Print and shaded views of the part. All mm, measured from the part's lowest x, y and z. A direction names the side the tool comes from. Give positions to 0.01 mm unless a question says otherwise; leave off trailing zeros. Loops run counter-clockwise (first coordinate to the right, second up) from the corner with the lowest first, then second, coordinate; pieces in that order, holes last. Notation, with made-up numbers: (39, 42) -> (79, 42) arc R24 ccw to (79, 80) -> close; hole circle Ø1 at (81, -18). An arc over 180 degrees is marked (long way). Write each question's results on one line, items separated by ' | '. Start each with the question number.
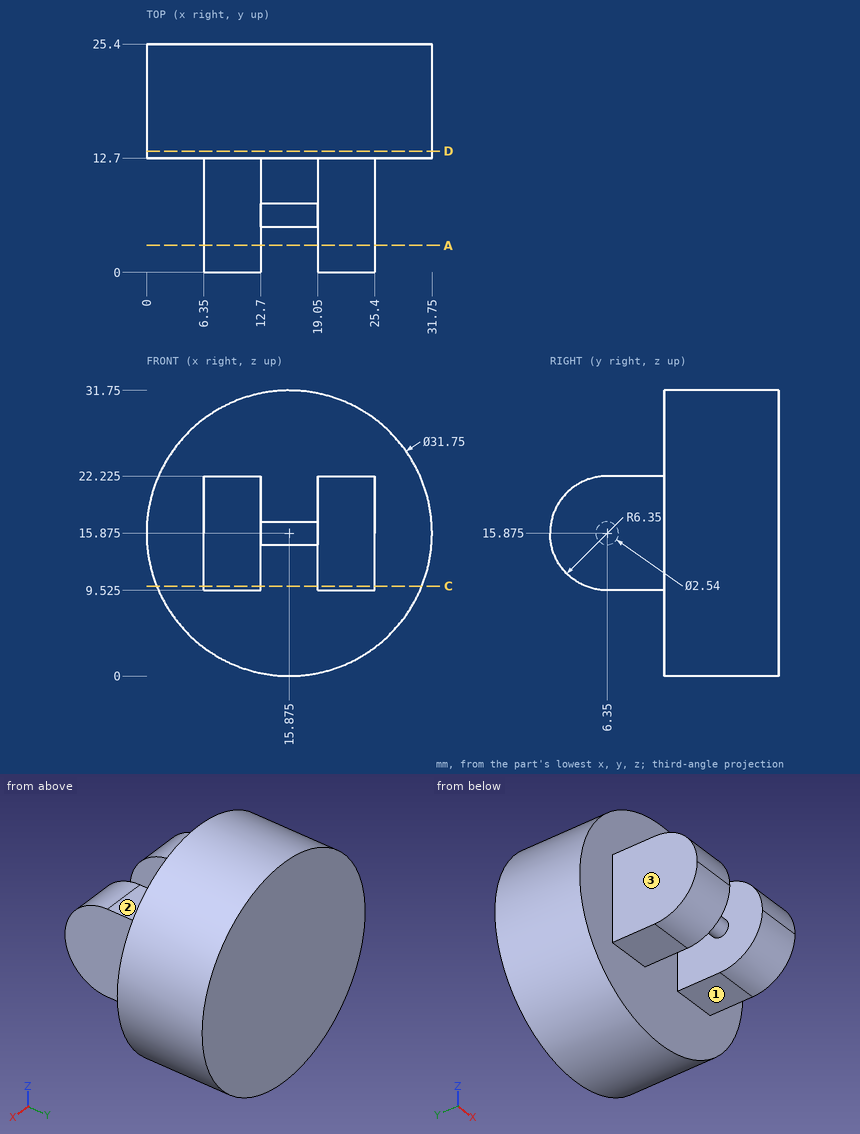
Q1. Saw through at A-A, the plane y = 3. List the corners of the cut face in (x, z), then the cut area to 3 significant figures.
Q2. Wall check: L1, parallel to Y at x = 9.5, z = 23.5; L2, parallel to X at y = 14, z = 16; L3, parallel to Z at x = 9.5, y = 8.75 (3 decimals). Give the ranges that are in metal, low to high.
Q3. Saw through at C-C, the plane z = 10. List the corners of the cut face in (x, y).
Q4. Which spindle directions (+Z, -Z, +X, -X, +Y, -Y) get a long thin tool onto all of the face, cutting with end or side? Do the marked faces 1, 2 and 3. Say none if no direction does.
Q5. Drop flat-ended pins along their axis: pin 1 (12 mm diameter, centred on x = 23.5, y = 22.5, fed in from -Z); pin 2 (1.9 mm diameter, centred on x = 21, y = 8, fed in from -Z) (3 decimals); pin 3 (7 mm diameter, centred on x = 10, y = 10.5, fed in from +Z). Give the stop position or say it passes through.
Q6. Saw through at D-D, the plane y = 13.5. List the corners of the cut face in (x, z) (3 decimals), then the cut area to 3 significant figures.
Answer block:
1) outline: (6.35, 10.48) -> (12.7, 10.48) -> (12.7, 21.27) -> (6.35, 21.27) -> close; (19.05, 10.48) -> (25.4, 10.48) -> (25.4, 21.27) -> (19.05, 21.27) -> close | area: 137 mm2
2) L1: y = 12.7 to 25.4 | L2: x = 0 to 31.75 | L3: z = 9.525 to 22.225
3) outline: (1.13, 12.7) -> (6.35, 12.7) -> (6.35, 3.94) -> (12.7, 3.94) -> (12.7, 12.7) -> (19.05, 12.7) -> (19.05, 3.94) -> (25.4, 3.94) -> (25.4, 12.7) -> (30.62, 12.7) -> (30.62, 25.4) -> (1.13, 25.4) -> close
4) face 1: -Z, +X, -X, -Y | face 2: +Z, +X, -X, -Y | face 3: +Z, -Z, -X, -Y
5) pin 1: stops at z = 0.08 | pin 2: stops at z = 9.525 | pin 3: stops at z = 31.43
6) outline: circle Ø31.75 at (15.875, 15.875) | area: 792 mm2
